Could you check a few things on this model? Use its own coordinates, in mm. A direction names the side the tool comes from. Coordinates: 2 decimals unless noted, no trailing zeros. Write each loop counter-clockwise with the first axis right and the second up, starting at its lowest first coordinate (ties: lowest second). Pieces come first, ordered by that corner, then holes.
Item 1: I want a section at C-C on y = -52. Please give me the cut outline in (x, z).
Item 2: I want a section at A-A on z = 8.25. Please give me the cut outline in (x, y).
Item 3: I want a section at B-B on x = 60. Please give me the cut outline in (y, z).
Item 4: If I drill on probe 1 along X at (y, z) = (-28, 1); probe 2 along X at (y, z) = (24, 12.25); probe 3 along X at (y, z) = (47.5, 8.5), over which ranges is the centre line in solid material (lowest first)?
Item 5: I want a section at D-D on x = -7. Please give me the cut outline in (y, z).
Item 6: Which directions (+Z, -Z, +X, -X, +Y, -Y) give clear straight access to the entire face, cutting with the end or side of a thin tool? Please do faces 1 (the flat face through (51, -8, 12.7)), 2 (the flat face through (58, 46.635, 6)), 3 (the flat face through (58, 49.175, 8)).
Item 7: For P1, Ø1.5, axis at x = -1, y = -53.5, coming from the +Z side, with a flat end and sliding along its axis, tell me the tip position at first contact or that it passes through.
Item 8: Thinking about a two-plate mould opening in X: for faces 4 (the flat face through (-39.86, -5, 8)), 5 (the flat face through (13, 59.335, 6)), 6 (the flat face through (76.98, -5, 6)), which applies, +X half, -X half, draft (parallel to the pull), parting line (faces both ways), or undercut?
from build123d import *

# Parameters (mm, degrees)
F0_W     = 127
F0_H     = 127
F0_W_2   = 12.7
F0_H_2   = 101.6
F1_DEPTH = 12.7
F2_T     = -2.54


with BuildPart() as f1:
    # F0 (on Top) → F1 (new body)
    with BuildSketch(Plane.XY):
        with Locations((13.4799859107, -4.1653172493)):
            Rectangle(F0_W, F0_H)
        with Locations((-30.9700140893, -4.1653172493)):
            Rectangle(F0_W_2, F0_H_2, mode=Mode.SUBTRACT)
        with Locations((57.9299859107, -4.1653172493)):
            Rectangle(F0_W_2, F0_H_2, mode=Mode.SUBTRACT)
    extrude(amount=F1_DEPTH)

    # F2
    f2_openings = [f1.faces().sort_by_distance(p)[0] for p in [
        (13.479986, -4.165317, 12.7),
    ]]
    offset(amount=F2_T, openings=f2_openings, kind=Kind.INTERSECTION)


solid = f1.part
Response values:
1. outline: (-50.02, 0) - (-37.32, 0) - (-37.32, 12.7) - (-39.86, 12.7) - (-39.86, 2.54) - (-47.48, 2.54) - (-47.48, 12.7) - (-50.02, 12.7) - close; (-24.62, 0) - (51.58, 0) - (51.58, 12.7) - (49.04, 12.7) - (49.04, 2.54) - (-22.08, 2.54) - (-22.08, 12.7) - (-24.62, 12.7) - close; (64.28, 0) - (76.98, 0) - (76.98, 12.7) - (74.44, 12.7) - (74.44, 2.54) - (66.82, 2.54) - (66.82, 12.7) - (64.28, 12.7) - close
2. outline: (-50.02, -67.67) - (76.98, -67.67) - (76.98, 59.33) - (-50.02, 59.33) - close; (-39.86, -57.51) - (-22.08, -57.51) - (-22.08, 49.17) - (-39.86, 49.17) - close; (49.04, -57.51) - (66.82, -57.51) - (66.82, 49.17) - (49.04, 49.17) - close; hole (-47.48, -65.13) - (74.44, -65.13) - (74.44, 56.79) - (-47.48, 56.79) - close; hole (-37.32, -54.97) - (-24.62, -54.97) - (-24.62, 46.63) - (-37.32, 46.63) - close; hole (51.58, -54.97) - (64.28, -54.97) - (64.28, 46.63) - (51.58, 46.63) - close
3. outline: (-67.67, 0) - (-54.97, 0) - (-54.97, 12.7) - (-57.51, 12.7) - (-57.51, 2.54) - (-65.13, 2.54) - (-65.13, 12.7) - (-67.67, 12.7) - close; (46.63, 0) - (59.33, 0) - (59.33, 12.7) - (56.79, 12.7) - (56.79, 2.54) - (49.17, 2.54) - (49.17, 12.7) - (46.63, 12.7) - close
4. probe 1: x = -50.02 to -37.32, -24.62 to 51.58, 64.28 to 76.98
4. probe 2: x = -50.02 to -47.48, -39.86 to -37.32, -24.62 to -22.08, 49.04 to 51.58, 64.28 to 66.82, 74.44 to 76.98
4. probe 3: x = -50.02 to -47.48, -39.86 to -22.08, 49.04 to 66.82, 74.44 to 76.98
5. outline: (-67.67, 0) - (59.33, 0) - (59.33, 12.7) - (56.79, 12.7) - (56.79, 2.54) - (-65.13, 2.54) - (-65.13, 12.7) - (-67.67, 12.7) - close
6. face 1: +Z, +X, -X, +Y, -Y
6. face 2: +Z, -Z
6. face 3: +Z
7. P1: stops at z = 2.54
8. face 4: undercut
8. face 5: draft
8. face 6: +X half
